from build123d import *

# Parameters (mm, degrees)
SKETCH1_R           = 1.275
BOSS_EXTRUDE1_DEPTH = 5
SKETCH2_W           = 9.1
SKETCH2_H           = 17.8
BOSS_EXTRUDE2_DEPTH = 20
BOSS_EXTRUDE3_DEPTH = 3
CUT_EXTRUDE1_DEPTH  = 15
SKETCH7_W           = 24.2
SKETCH7_H           = 42.2
BOSS_EXTRUDE4_DEPTH = 5
SKETCH8_R           = 12
CUT_EXTRUDE3_DEPTH  = 5
SKETCH10_W          = 48.2
SKETCH10_H          = 17.8
BOSS_EXTRUDE5_DEPTH = 5
FILLET1_R           = 3
BOSS_EXTRUDE6_START = 6.1
BOSS_EXTRUDE6_DEPTH = 6.1
SKETCH13_R          = 2.6
CUT_EXTRUDE4_DEPTH  = 16
FILLET2_R           = 3
SKETCH14_W          = 25
SKETCH14_H          = 48.2
BOSS_EXTRUDE7_DEPTH = 5


with BuildPart() as part:
    # Sketch1 → Boss-Extrude1 (new body)
    # profile 1 of 2: a face of its own
    with BuildSketch(Plane(origin=(0, 0, 0), x_dir=(0, 0, -1), z_dir=(1, 0, 0))):
        Polygon((-4.381647728, -34.17856484), (-0.382647728, -30.17956484), (-0.382647728, 8.02143516), (-6.482647728, 8.02143516), (-9.382647728, 8.02143516), (-9.382647728, -34.17856484), align=None)
        with Locations((-5.982647728, 2.42143516)):
            Circle(SKETCH1_R, mode=Mode.SUBTRACT)
        with Locations((-5.982647728, -28.57856484)):
            Circle(SKETCH1_R, mode=Mode.SUBTRACT)
    # profile 2 of 2: a face of its own
    with BuildSketch(Plane(origin=(0, 0, 0), x_dir=(0, 0, -1), z_dir=(1, 0, 0))):
        Polygon((2.617352272, 8.02143516), (2.617352272, 25.82143516), (-6.482647728, 25.82143516), (-6.482647728, 8.02143516), (-0.382647728, 8.02143516), align=None)
    extrude(amount=BOSS_EXTRUDE1_DEPTH)

    # Sketch2 → Boss-Extrude2 (add)
    with BuildSketch(Plane(origin=(5, 0, 0), x_dir=(0, 0, -1), z_dir=(1, 0, 0))):
        with Locations((-1.932647728, 16.92143516)):
            Rectangle(SKETCH2_W, SKETCH2_H)
    extrude(amount=BOSS_EXTRUDE2_DEPTH)

    # Sketch3 → Boss-Extrude3 (add)
    with BuildSketch(Plane(origin=(0, 0, 0.382647728), x_dir=(-1, 0, 0), z_dir=(0, 0, -1))):
        Polygon((-25, 8.02143516), (0, 8.02143516), (0, -30.17956484), (-5, -30.17956484), align=None)
    extrude(amount=BOSS_EXTRUDE3_DEPTH)

    # Sketch4 → Cut-Extrude1 (cut, symmetric)
    with BuildSketch(Plane(origin=(5, 0, 0), x_dir=(0, 0, -1), z_dir=(1, 0, 0))):
        Polygon((-0.382647728, -30.17956484), (2.617352272, -27.17956484), (2.617352272, -30.17956484), align=None)
    extrude(amount=CUT_EXTRUDE1_DEPTH, both=True, mode=Mode.SUBTRACT)


with BuildPart() as body_2:
    # Mirror14: mirrored copy
    add(part.part.mirror(Plane.XY.offset(21.482647728)))


with BuildPart() as part_1:
    add(part.part)

    add(body_2.part)  # Boss-Extrude4 merges body 2
    # Sketch7 → Boss-Extrude4 (add)
    with BuildSketch(Plane(origin=(5, 0, 0), x_dir=(0, 0, -1), z_dir=(1, 0, 0))):
        with Locations((-21.482647728, -13.07856484)):
            Rectangle(SKETCH7_W, SKETCH7_H)
    extrude(amount=-BOSS_EXTRUDE4_DEPTH)

    # Sketch8 → Cut-Extrude3 (cut)
    with BuildSketch(Plane(origin=(5, 0, 0), x_dir=(0, 0, -1), z_dir=(1, 0, 0))):
        with Locations((-21.482647728, -13.07856484)):
            Circle(SKETCH8_R)
    extrude(amount=-CUT_EXTRUDE3_DEPTH, mode=Mode.SUBTRACT)

    # Sketch10 → Boss-Extrude5 (add)
    with BuildSketch(Plane(origin=(25, 0, 0), x_dir=(0, 0, -1), z_dir=(1, 0, 0))):
        with Locations((-21.482647728, 16.92143516)):
            Rectangle(SKETCH10_W, SKETCH10_H)
    extrude(amount=-BOSS_EXTRUDE5_DEPTH)

    # Fillet1
    fillet1_edges = [part_1.edges().sort_by_distance(p)[0] for p in [
        (20, 16.92143516, 36.482647728),
        (20, 16.92143516, 6.482647728),
    ]]
    fillet(fillet1_edges, radius=FILLET1_R)

    # Sketch12 → Boss-Extrude6 (add)
    with BuildSketch(Plane(origin=(0, 25.82143516, 0), x_dir=(1, 0, 0), z_dir=(0, 1, 0)).offset(BOSS_EXTRUDE6_START)):
        with BuildLine():
            Line((25, 2.617352272), (0, 2.617352272))
            Line((0, 2.617352272), (0, -6.482647728))
            Line((0, -6.482647728), (17, -6.482647728))
            ThreePointArc((17, -6.482647728), (19.121320344, -7.361327384), (20, -9.482647728))
            Line((20, -9.482647728), (20, -33.482647728))
            ThreePointArc((20, -33.482647728), (19.121320344, -35.603968072), (17, -36.482647728))
            Line((17, -36.482647728), (0, -36.482647728))
            Line((0, -36.482647728), (0, -45.582647728))
            Line((0, -45.582647728), (25, -45.582647728))
            Line((25, -45.582647728), (25, 2.617352272))
        make_face()
    extrude(amount=-BOSS_EXTRUDE6_DEPTH)

    # Sketch13 → Cut-Extrude4 (cut)
    with BuildSketch(Plane.ZY.offset(-20)):
        with Locations((29.482647728, 16.92143516)):
            Circle(SKETCH13_R)
        with Locations((13.482647728, 16.92143516)):
            Circle(SKETCH13_R)
    extrude(amount=-CUT_EXTRUDE4_DEPTH, mode=Mode.SUBTRACT)

    # Fillet2
    # the kernel refuses this fillet: 3 mm, written as the material it adds along each edge
    with BuildSketch(Plane(origin=(0, 8.02143516, 6.482647728), x_dir=(0, 1, 0), z_dir=(1, 0, 0)), Plane(origin=(0, 8.02143516, 36.482647728), x_dir=(0, 0, -1), z_dir=(1, 0, 0))) as fillet2_piece_1:
        with BuildLine():
            CenterArc((FILLET2_R, FILLET2_R), FILLET2_R, 180, 90)
            Line((0, FILLET2_R), (0, 0))
            Line((0, 0), (FILLET2_R, 0))
        make_face()
    extrude(amount=5)

    # Sketch14 → Boss-Extrude7 (add)
    with BuildSketch(Plane(origin=(0, 31.92143516, 0), x_dir=(1, 0, 0), z_dir=(0, 1, 0))):
        with Locations((12.5, -21.482647728)):
            Rectangle(SKETCH14_W, SKETCH14_H)
    extrude(amount=-BOSS_EXTRUDE7_DEPTH)


solid = part_1.part
Geometry check sheet. Reference: the model listing, model coordinates, mm. A direction names the side the tool comes from. Round coordinates to 2 decimals unless told otherwise and drop trailing zeros. Write each loop counter-clockwise with the first axis right and the second up, starting at its lowest first coordinate (ties: lowest second). Pieces come first, ordered by that corner, then holes. Notation, with made-up numbers: (84.5, 6) - (124.5, 6) arc R28 ccw to (124.5, 27) - close; hole circle Ø8 at (-39, 19). An arc over 180 degrees is marked (long way). One line per item, written item: value.
1. Cross-section at A-A on y = 22. Record the boundary of the cut face in (x, z).
The answers:
outline: (0, -2.62) - (25, -2.62) - (25, 45.58) - (0, 45.58) - (0, 36.48) - (17, 36.48) arc R3 cw to (20, 33.48) - (20, 9.48) arc R3 cw to (17, 6.48) - (0, 6.48) - close
2. Mould release check, pull along Z, two halves, no side actions. Record for faces 4 (the face through (10, 9, -2.617)), 5 (the face through (25, 20, 22)), 6 (the face through (13, -7, 0.383)): released by +Z, released by -Z, zero draft, split by the parting line, or undercut.
The answers:
face 4: released by -Z
face 5: zero draft
face 6: undercut
3. Cross-section at D-D on z = 21.5. Record the boundary of the cut face in (x, y).
The answers:
outline: (0, -34.18) - (5, -34.18) - (5, -25.08) - (0, -25.08) - close; (0, -1.08) - (5, -1.08) - (5, 8.02) - (0, 8.02) - close; (0, 26.92) - (20, 26.92) - (20, 8.02) - (25, 8.02) - (25, 31.92) - (0, 31.92) - close
4. Set-up check for faces 1 (the face through (22, 8.021, 21)), 2 (the face through (12, 31.921, 21)), 3 (the face through (2.465, 8.924, 35.627)): record each of +Z, -Z, +X, -X, +Y, -Y from which the full face is reachable in a straight line by a thin tool's end or side.
The answers:
face 1: +X, -Y
face 2: +Z, -Z, +X, -X, +Y
face 3: -X
5. Cross-section at C-C on x = 21.75. Record the boundary of the cut face in (y, z).
The answers:
outline: (1.81, -2.62) - (31.92, -2.62) - (31.92, 45.58) - (1.81, 45.58) - (1.81, 42.58) - (8.02, 42.58) - (8.02, 0.38) - (1.81, 0.38) - close; hole circle Ø5.2 at (16.92, 13.48); hole circle Ø5.2 at (16.92, 29.48)
6. Cross-section at B-B on z = 8. Record the boundary of the cut face in (x, y), and give its area (3 significant figures).
The answers:
outline: (0, -34.18) - (5, -34.18) - (5, 8.41) - (0, 8.41) - close; (0, 26.92) - (19.61, 26.92) - (19.61, 8.02) - (25, 8.02) - (25, 31.92) - (0, 31.92) - close
area: 440 mm^2
7. Depth check by flat-ended pin: pin 1 Ø3 at (y, z) = (16.92, 13.48) entering from -X; pin 2 Ø6 at (x, z) = (16, 13) entering from -Y; pin 3 Ø21 at (y, z) = (-21.5, 31) entering from +X; pin 4 Ø9.5 at (y, z) = (16.5, 26.5) entering from -X. Enter the tip coordinate at first touch or a pass-through.
The answers:
pin 1: passes through
pin 2: stops at y = 26.92
pin 3: stops at x = 5
pin 4: stops at x = 20
8. Scan lines: L1, parallel to Z at x = 11.75, y = 25; L2, parallel to Y at x = 3.25, z = 22; L3, parallel to Z at x = 8, y = -23. Record each from-to range of solid material in increasing order.
The answers:
L1: z = -2.62 to 6.48, 36.48 to 45.58
L2: y = -34.18 to -25.07, -1.09 to 8.02, 26.92 to 31.92
L3: z = -2.62 to 0.38, 42.58 to 45.58
